Source: CAD feature listing. Evaluate the final solid. Frame: model axes, mm. Round coordinates to 2 decimals unless told otherwise and drop trailing zeros. Loops run counter-clockwise (first coordinate to the right, second up) from the corner with the lowest first, then second, coordinate; pieces in that order, holes last. Notation, with made-up numbers: (63.5, 42.25) - (75.5, 42.25) arc R22 cw to (75.5, 59.25) - close; hole circle Ø5 at (40.5, -26.5). An arc over 180 degrees is marked (long way). Write item = value, one per line. Start each with the question number.
from build123d import *

# Parameters (mm, degrees)
BOSS_EXTRUDE1_DEPTH = 3
SKETCH2_R           = 1.75
CUT_EXTRUDE1_DEPTH  = 10
SKETCH3_R           = 1.75
CUT_EXTRUDE2_DEPTH  = 10


with BuildPart() as part:
    # Sketch1 → Boss-Extrude1 (new body)
    with BuildSketch(Plane(origin=(0, 0, 0), x_dir=(1, 0, 0), z_dir=(0, 1, 0))):
        Polygon((-150, 29.5), (0, 29.5), (0, 23), (-150, 23), (-150, 19.5), (0, 19.5), (0, 13), (-150, 13), (-150, 0), (0, 0), (100, 0), (100, 70), (-50, 70), (-150, 70), (-150, 54.5), (0, 54.5), (0, 48), (-150, 48), (-150, 44.5), (0, 44.5), (0, 38), (-150, 38), align=None)
    extrude(amount=BOSS_EXTRUDE1_DEPTH)

    # Sketch2 → Cut-Extrude1 (cut)
    with BuildSketch(Plane(origin=(0, 3, 0), x_dir=(1, 0, 0), z_dir=(0, 1, 0))):
        with Locations(Location((-145, 65, 0), (0, 0, 270))):
            Circle(SKETCH2_R)
        with Locations(Location((-135, 65, 0), (0, 0, 270))):
            Circle(SKETCH2_R)
        with Locations(Location((20, 65, 0), (0, 0, 270))):
            Circle(SKETCH2_R)
        with Locations(Location((30, 65, 0), (0, 0, 270))):
            Circle(SKETCH2_R)
    cut_extrude1 = extrude(amount=-CUT_EXTRUDE1_DEPTH, mode=Mode.SUBTRACT)

    # Sketch3 → Cut-Extrude2 (cut)
    with BuildSketch(Plane(origin=(0, 3, 0), x_dir=(1, 0, 0), z_dir=(0, 1, 0))):
        with Locations(Location((95, 65, 0), (0, 0, 270))):
            Circle(SKETCH3_R)
        with Locations(Location((90, 65, 0), (0, 0, 270))):
            Circle(SKETCH3_R)
    cut_extrude2 = extrude(amount=-CUT_EXTRUDE2_DEPTH, mode=Mode.SUBTRACT)

    # Mirror1: Cut-Extrude1, Cut-Extrude2 across plane
    add(cut_extrude1.mirror(Plane(origin=(0, 0, -35), x_dir=(1, 0, 0), z_dir=(0, 0, -1))), mode=Mode.SUBTRACT)
    add(cut_extrude2.mirror(Plane(origin=(0, 0, -35), x_dir=(1, 0, 0), z_dir=(0, 0, -1))), mode=Mode.SUBTRACT)


solid = part.part
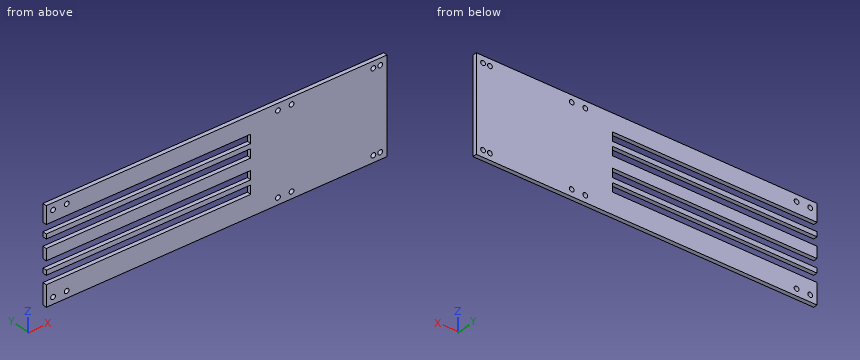
(1) Cut plane A-A (x = -56). Output: boundary loops of the cut face in (y, z).
(2) Material intervals for line 1 along Z through (x, y) = (-81.5, 1.15); line 2 along Z through (x, y) = (90, 1.7); line 3 along X through (y, z) = (0.9, -18), sorted ascending. Write a range as from..to.
(3) Cut plane B-B (y = 1.4). State how many separate pieces and enclosed holes the cut face has, and give its area (3 significant figures).
(4) Pin query (flat end, axial travel): P1, Ø1.5, axis at y = 1, z = -51.5, coming from the -X side. Return the tip coordinate at first contact, or that it passes through.
Solution:
q1.outline = (0, -70) - (3, -70) - (3, -54.5) - (0, -54.5) - close; (0, -48) - (3, -48) - (3, -44.5) - (0, -44.5) - close; (0, -38) - (3, -38) - (3, -29.5) - (0, -29.5) - close; (0, -23) - (3, -23) - (3, -19.5) - (0, -19.5) - close; (0, -13) - (3, -13) - (3, 0) - (0, 0) - close
q2.line_1 = -70..-54.5, -48..-44.5, -38..-29.5, -23..-19.5, -13..0
q2.line_2 = -70..-66.75, -63.25..-6.75, -3.25..0
q2.line_3 = 0..100
q3.separate_pieces = 1
q3.enclosed_holes = 12
q3.area = 13,500 mm^2
q4.P1 = 0
